CAD build for the part. Positions are in the model's coordinates, mm. Round coordinates to 2 decimals unless told otherwise and drop trailing zeros. Loops run counter-clockwise (first coordinate to the right, second up) from the corner with the lowest first, then second, coordinate; pieces in that order, holes last. Notation, with made-up numbers: M 20,-30 L 75,-30 A21 cw 75,-16 Z; hole C -36,26.5 d7. An arc over 180 degrees is marked long. One line per item, written item: value. Start each with the question number.
from build123d import *

# Parameters (mm, degrees)
SKETCH_1_R               = 1.5
EXTRUDE_1_DEPTH          = 8
CUT_EXTRUDE_1_DEPTH      = 1
CUT_EXTRUDE_1_DEPTH_BACK = 9
SKETCH_3_R               = 2.5
CUT_EXTRUDE_2_DEPTH      = 1
CUT_EXTRUDE_2_DEPTH_BACK = 9


with BuildPart() as part:
    # 草图1 → 凸台-拉伸1 (new body)
    with BuildSketch(Plane(origin=(0, 0, 0), x_dir=(1, 0, 0), z_dir=(0, 1, 0))):
        with BuildLine():
            Line((0, 19.5), (127.428932188, 19.5))
            ThreePointArc((127.428932188, 19.5), (132.048329851, 16.413417162), (130.964466094, 10.964466094))
            Line((130.964466094, 10.964466094), (103.428932188, -16.571067812))
            ThreePointArc((103.428932188, -16.571067812), (100.1846987, -18.738795325), (96.357864376, -19.5))
            Line((96.357864376, -19.5), (0, -19.5))
            ThreePointArc((0, -19.5), (-19.5, 0), (0, 19.5))
        make_face()
        with Locations((-5.656854249, 5.656854249)):
            Circle(SKETCH_1_R, mode=Mode.SUBTRACT)
        with Locations((5.656854249, 5.656854249)):
            Circle(SKETCH_1_R, mode=Mode.SUBTRACT)
        with Locations((5.656854249, -5.656854249)):
            Circle(SKETCH_1_R, mode=Mode.SUBTRACT)
        with Locations((-5.656854249, -5.656854249)):
            Circle(SKETCH_1_R, mode=Mode.SUBTRACT)
    extrude(amount=EXTRUDE_1_DEPTH)

    # 草图2 → 切除-拉伸1 (cut, two sides)
    with BuildSketch(Plane(origin=(0, 8, 0), x_dir=(1, 0, 0), z_dir=(0, 1, 0))) as cut_extrude_1_sk:
        with BuildLine():
            Line((73.487806691, -4.085786438), (83.902020254, 6.328427125))
            ThreePointArc((83.902020254, 6.328427125), (85.199713649, 7.19551813), (86.730447378, 7.5))
            Line((86.730447378, 7.5), (105.701010127, 7.5))
            ThreePointArc((105.701010127, 7.5), (107.548769192, 6.265366865), (107.115223689, 4.085786438))
            Line((107.115223689, 4.085786438), (96.701010127, -6.328427125))
            ThreePointArc((96.701010127, -6.328427125), (95.403316732, -7.19551813), (93.872583002, -7.5))
            Line((93.872583002, -7.5), (74.902020254, -7.5))
            ThreePointArc((74.902020254, -7.5), (73.054261189, -6.265366865), (73.487806691, -4.085786438))
        make_face()
    extrude(amount=CUT_EXTRUDE_1_DEPTH, mode=Mode.SUBTRACT)
    extrude(cut_extrude_1_sk.sketch, amount=-CUT_EXTRUDE_1_DEPTH_BACK, mode=Mode.SUBTRACT)

    # 草图3 → 切除-拉伸2 (cut, two sides)
    with BuildSketch(Plane(origin=(0, 8, 0), x_dir=(1, 0, 0), z_dir=(0, 1, 0))) as cut_extrude_2_sk:
        with Locations((58.002525317, -12.5)):
            Circle(SKETCH_3_R)
        with Locations((83.002525317, 12.5)):
            Circle(SKETCH_3_R)
        with Locations((97.600505063, -12.5)):
            Circle(SKETCH_3_R)
        with Locations((122.600505063, 12.5)):
            Circle(SKETCH_3_R)
    extrude(amount=CUT_EXTRUDE_2_DEPTH, mode=Mode.SUBTRACT)
    extrude(cut_extrude_2_sk.sketch, amount=-CUT_EXTRUDE_2_DEPTH_BACK, mode=Mode.SUBTRACT)


solid = part.part
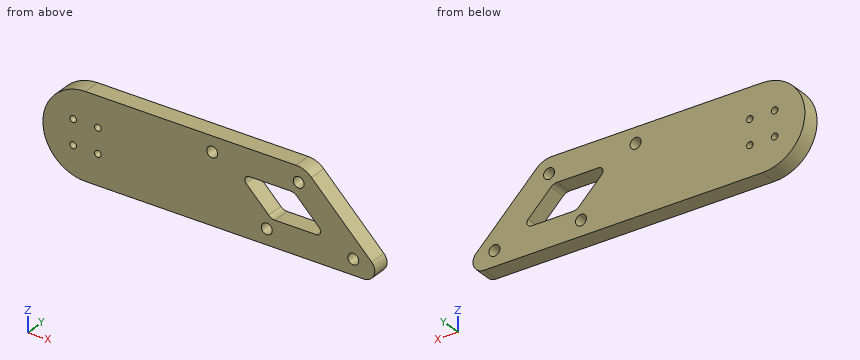
(1) Slice it at A-A, the plane z = 0. List the corners of the cut face in (x, y), and give its area (3 significant figures).
(2) Flat gauge pins, fed straight in: P1, Ø1, axis at y = 4, z = -7, coming from the +X side; P2, Ø1, axis at y = 1, z = 2.5, coming from the -X side. Where does each tip first touch, or does it go through?
(3) Probe L1, parallel to X at y = 5.75, z = -10.5; L2, parallel to X at y = 3.25, z = 12.5; L3, parallel to Z at x = -7, y = 3.25. List the from-to ranges inside material, lowest first.
(4) Slice it at C-C, the plane y = 1.25. Count the separate pieces of the cut face and the enclosed holes in it, and give its area (3 significant figures).
(5) Slice it at B-B, the plane z = -12.5. List the corners of the cut face in (x, y), and give its area (3 significant figures).
Check result:
1. outline: M -19.5,0 L 77.57,0 L 77.57,8 L -19.5,8 Z; M 103.03,0 L 120,0 L 120,8 L 103.03,8 Z
1. area: 912 mm^2
2. P1: stops at x = 127.5
2. P2: stops at x = -19.4
3. L1: x = -16.43 to 81.5, 84.5 to 121.1, 124.1 to 130.5
3. L2: x = -14.97 to 55.5, 60.5 to 95.1, 100.1 to 107.5
3. L3: z = -18.2 to -6.32, -4.99 to 4.99, 6.32 to 18.2
4. separate pieces: 1
4. enclosed holes: 9
4. area: 4,770 mm^2
5. outline: M -14.97,0 L 80.5,0 L 80.5,8 L -14.97,8 Z; M 85.5,0 L 120.1,0 L 120.1,8 L 85.5,8 Z; M 125.1,0 L 132.01,0 L 132.01,8 L 125.1,8 Z
5. area: 1,100 mm^2
